Check sheet for the drawn part. Datum: minimum x, y, z corner. Units: mm. A direction names the side the tool comes from. Round coordinates to 2 decimals unless told otherwise and drop trailing zeros. Write each loop counter-clockwise with the first axis right and the second up, starting at its lowest first coordinate (ties: lowest second). Pieces come first, ordered by that corner, then holes. Notation, with made-up numbers: (29.5, 52) - (63.5, 52) arc R10 ccw to (63.5, 56) - close; hole circle Ø7 at (13.25, 38). An arc over 180 degrees is marked (long way). Write each question's results on one line, items separated by ' | '.
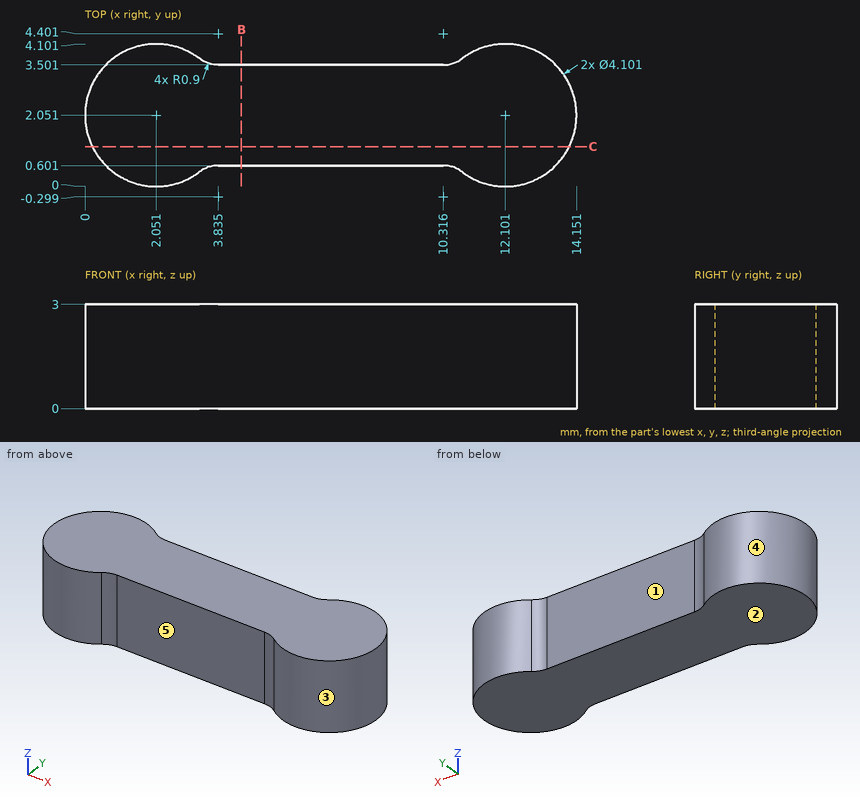
(1) Go/stop test with flat-tipped pins: pin 1 Ø1 at (y, z) = (3.5, 1.5) entering from +X; pin 2 Ø1 at (x, z) = (6.5, 0.5) entering from +Y; pin 3 Ø0.9 at (x, z) = (6, 1.5) entering from -Y. Record where each tip stops, or that it passes through.
Answer:
pin 1: x = 13.92 | pin 2: y = 3.5 | pin 3: y = 0.6
(2) Thickness scan on L1, parallel to X at y = 0.4, z = 2.2 (1 decimal); L2, parallel to X at y = 0.5, z = 1.8 (1 decimal); L3, parallel to Y at x = 8.5, z = 1. Record the ranges inside material, lowest first.
Answer:
L1: 0.8 to 3.3, 10.9 to 13.3 | L2: 0.7 to 3.4, 10.7 to 13.4 | L3: 0.6 to 3.5
(3) Set-up check for the marked faces 4 and 5: record each of +Z, -Z, +X, -X, +Y, -Y from which the full face is reachable in a straight line by a thin tool's end or side.
Answer:
face 4: +Z, -Z | face 5: +Z, -Z, -Y
(4) Mould release check, pull along X, two halves, no side actions. Record for the marked faces 1, 2 and 3: released by +X, released by -X, zero draft, split by the parting line, or undercut.
Answer:
face 1: undercut | face 2: zero draft | face 3: undercut
(5) Section check B-B (x = 4.5). Record the cut outline in (y, z).
Answer:
outline: (0.6, 0) - (3.5, 0) - (3.5, 3) - (0.6, 3) - close
(6) Section check C-C (y = 1.15). Record the cut outline in (x, z).
Answer:
outline: (0.21, 0) - (13.94, 0) - (13.94, 3) - (0.21, 3) - close
